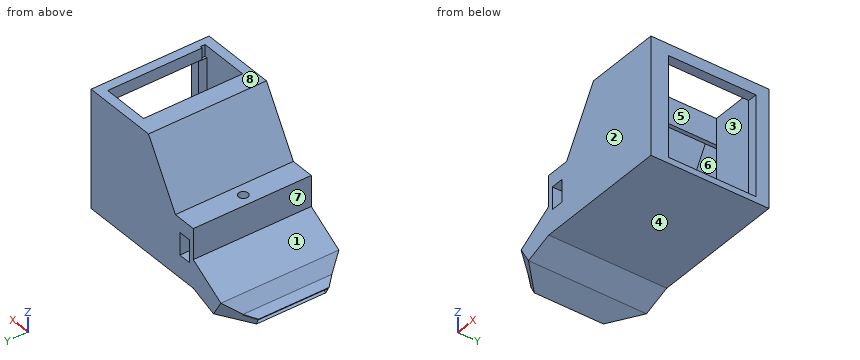
```python
from build123d import *

# Parameters (mm, degrees)
F0_W      = 5.5
F0_H      = 9.5
F1_DEPTH  = 50
F2_T      = -2.5
F3_W      = 46
F3_H      = 4
F4_DEPTH  = 18
F5_DEPTH  = 30
F6_W      = 2
F6_H      = 3
F7_DEPTH  = 42.640873421
F8_W      = 20
F8_H      = 42
F9_DEPTH  = 4.859126579
F10_W     = 1.7037652433
F10_H     = 3.2813884318
F11_DEPTH = 45
F12_W     = 1
F12_H     = 2
F13_DEPTH = 5
F14_DEPTH = 42.640873421
F15_DEPTH = 5
F16_DEPTH = 3
F17_DEPTH = 2
F20_DEPTH = 50
F21_DEPTH = 25
F22_DEPTH = 15
F23_DEPTH = 0.5
F24_DEPTH = 3
F25_DEPTH = 2
F26_R     = 2
F27_DEPTH = 6


with BuildPart() as f1:
    # F0 (on Front) → F1 (new body)
    with BuildSketch(Plane.XZ):
        Polygon((0, 12), (0, 0), (20, 0), (20, 25), (10, 25), (0, 25), align=None)
        with Locations((4.75, 14.25)):
            Rectangle(F0_W, F0_H, mode=Mode.SUBTRACT)
        Polygon((20, 25), (20, 0), (25, 0), (25, 50), (10, 25), align=None)
        Polygon((-11.2763114494, -4.1042417199), (0, 0), (0, 12), (-15.3952030634, 2.7539454948), align=None)
    extrude(amount=F1_DEPTH)

    # F2
    f2_openings = [f1.faces().sort_by_distance(p)[0] for p in [
        (25, -25, 25),
    ]]
    offset(amount=F2_T, openings=f2_openings, kind=Kind.INTERSECTION)

    # F3 (on face) → F4 (cut)
    with BuildSketch(Plane(origin=(-10.0986787248, 0, -6.0650667312), x_dir=(0, -1, 0), z_dir=(-0.8572734018, 0, -0.5148614518))):
        with Locations((25, 6.2872808221)):
            Rectangle(F3_W, F3_H)
    extrude(amount=-F4_DEPTH, mode=Mode.SUBTRACT)

    # F5 (add): a face of the model
    f5_faces = [f1.faces().sort_by_distance(p)[0] for p in [
        (25, -25, 0.7071067812),
    ]]
    extrude(f5_faces, amount=F5_DEPTH)

    # F6 (on face) → F7 (join, through all)
    with BuildSketch(Plane(origin=(0, 0, 45.140873421), x_dir=(1, 0, 0), z_dir=(0, 0, -1))):
        with Locations((54, 46)):
            Rectangle(F6_W, F6_H)
        with Locations((54, 4)):
            Rectangle(F6_W, F6_H)
    extrude(amount=F7_DEPTH)

    # F8 (on face) → F9 (cut, through all)
    with BuildSketch(Plane.XY.offset(50)):
        with Locations((43, -25)):
            Rectangle(F8_W, F8_H)
    extrude(amount=-F9_DEPTH, mode=Mode.SUBTRACT)

    # F10 (on face) → F11 (join, through all)
    with BuildSketch(Plane.XZ.offset(2.5)):
        with Locations((32.1481173784, 43.5001792051)):
            Rectangle(F10_W, F10_H)
    extrude(amount=F11_DEPTH)

    # F12 (on face) → F13 (cut)
    with BuildSketch(Plane.XY.offset(50)):
        with Locations((53.5, -45)):
            Rectangle(F12_W, F12_H)
    extrude(amount=-F13_DEPTH, mode=Mode.SUBTRACT)

    # F14 (add, through all): faces of the model
    f14_faces = [f1.faces().sort_by_distance(p)[0] for p in [
        (43, -46.75, 45.140873421),
        (43, -3.25, 45.140873421),
    ]]
    extrude(f14_faces, amount=F14_DEPTH)

    # F15 (add): a face of the model
    f15_faces = [f1.faces().sort_by_distance(p)[0] for p in [
        (55, -25, 0.7071067812),
    ]]
    extrude(f15_faces, amount=F15_DEPTH)

    # F16 (add): a face of the model
    f16_faces = [f1.faces().sort_by_distance(p)[0] for p in [
        (32.1481173784, -25, 41.8594849892),
    ]]
    extrude(f16_faces, amount=F16_DEPTH)

    # F17 (add): a face of the model
    f17_faces = [f1.faces().sort_by_distance(p)[0] for p in [
        (56.5014165477, -44.5, 23.810402831),
    ]]
    extrude(f17_faces, amount=F17_DEPTH)

    # F19 (on face) → F20 (join)
    with BuildSketch(Plane.XZ.offset(50)):
        Polygon((-11.2763114494, -4.1042417199), (-15.3952030634, 2.7539454948), (-19.6083863192, -2.1957097309), (-23.1083863192, -3.9201829974), (-21.6654660693, -6.8880073104), align=None)
    extrude(amount=-F20_DEPTH)

    # F18 (on face) → F21 (cut)
    with BuildSketch(Plane(origin=(-5.2965243386, 0, 8.819012226), x_dir=(0.8572734018, 0, 0.5148614518), z_dir=(-0.5148614518, 0, 0.8572734018))):
        Polygon((-33.7799977267, -50), (-11.7799977267, -50), (-33.7799977267, -28), align=None)
        Polygon((-33.7799977267, -22), (-11.7799977267, 0), (-33.7799977267, 0), align=None)
    extrude(amount=-F21_DEPTH, mode=Mode.SUBTRACT)

    # F22 (cut): a face of the model
    f22_faces = [f1.faces().sort_by_distance(p)[0] for p in [
        (-22.3892898276, -25, -5.3992335904),
    ]]
    extrude(f22_faces, amount=-F22_DEPTH, mode=Mode.SUBTRACT)

    # F23 (add): a face of the model
    f23_faces = [f1.faces().sort_by_distance(p)[0] for p in [
        (-21.2912627093, -25, -3.0248741153),
    ]]
    extrude(f23_faces, amount=-F23_DEPTH)

    # F24 (cut): a face of the model
    f24_faces = [f1.faces().sort_by_distance(p)[0] for p in [
        (60, -25, 0.7071067812),
    ]]
    extrude(f24_faces, amount=-F24_DEPTH, mode=Mode.SUBTRACT)

    # F25 (add): a face of the model
    f25_faces = [f1.faces().sort_by_distance(p)[0] for p in [
        (6.25, -25, 21.5),
    ]]
    extrude(f25_faces, amount=F25_DEPTH)

    # F26 (on face) → F27 (cut)
    with BuildSketch(Plane.XY.offset(25)):
        with Locations((5, -25)):
            Circle(F26_R)
    extrude(amount=-F27_DEPTH, mode=Mode.SUBTRACT)


solid = f1.part
```
The listing builds one solid part. Answer for the finished solid, in the listing's coordinates (mm). Face numbers are marked on the shaded views. A direction names the side the tool comes from. Coordinates: 2 decimals unless noted, no trailing zeros. Write each loop counter-clockwise with the first axis right and the second up, starting at its lowest first coordinate (ties: lowest second). Pieces come first, ordered by that corner, then holes. Notation, with made-up numbers: (83.5, -25.75) -> (94.5, -25.75) arc R32 cw to (94.5, 11.25) -> close; hole circle Ø10 at (75.5, -6.5). An arc over 180 degrees is marked (long way). Write each question's results on one line, items separated by ' | '. Start each with the question number.
1) For a pull along X with two mould halves and no side action, classify the marked faces 1, 2 and 3 as +X half, -X half, draft (parallel to the pull), parting line (faces both ways), or undercut.
2) Straight lines are drawn through the part: probe 1 along Y at (x, z) = (5, 22); probe 2 along Y at (x, z) = (47, 23.5); probe 3 along Z at (x, y) = (32, -18.5). For each, find the intervals that lie inside material, in ascending order.
3) A cutting plane is placed at B-B (x = 42). Determine the outline of the cut face in (y, z).
4) Flat-ended cylindrical pins translate along their axes: pin 1 Ø1.5 at (y, z) = (-15, 20.5) entering from +X; pin 2 Ø10.5 at (y, z) = (-23, 15.5) entering from -X; pin 3 Ø3 at (x, y) = (3.5, -13.5) entering from +Z. Find the tip coordinate at first contact, or state that the pin passes through.
5) A tool of negligible diameter and unlimited length cuts with its end or side. For the marked faces 4, 5, 6, 7 and 8, from which of +Z, -Z, +X, -X, +Y, -Y can it reach the whole face along a straight path? Write none if from no direction.
6) A cutting plane is placed at C-C (y = -41.5). Count the separate pieces of the cut face and the enclosed holes in it, then the cut area to 3 significant figures.
7) A cutting plane is placed at D-D (x = 20.5). Determine the outline of the cut face in (y, z), then the cut area to 3 significant figures.
8) A cutting plane is placed at A-A (x = 5). Determine the outline of the cut face in (y, z).
Values follow:
1) face 1: -X half | face 2: draft | face 3: undercut
2) probe 1: -50 to -27, -23 to 0 | probe 2: -50 to -46, -4 to 0 | probe 3: 0 to 2.5, 38.86 to 50
3) outline: (-50, 0) -> (0, 0) -> (0, 50) -> (-4, 50) -> (-4, 2.5) -> (-46, 2.5) -> (-46, 50) -> (-50, 50) -> close
4) pin 1: x = 10 | pin 2: x = -2.91 | pin 3: z = 25
5) face 4: -Z, +X, +Y, -Y | face 5: +Z | face 6: none | face 7: +Z, -X, +Y, -Y | face 8: +Z, +X, -X, +Y, -Y
6) separate pieces: 2 | enclosed holes: 1 | area: 516 mm²
7) outline: (-50, 0) -> (0, 0) -> (0, 42.5) -> (-50, 42.5) -> close; hole (-47.5, 2.5) -> (-2.5, 2.5) -> (-2.5, 37.64) -> (-47.5, 37.64) -> close | area: 544 mm²
8) outline: (-50, 0) -> (0, 0) -> (0, 9.5) -> (-50, 9.5) -> close; (-50, 19) -> (-27, 19) -> (-27, 25) -> (-50, 25) -> close; (-23, 19) -> (0, 19) -> (0, 25) -> (-23, 25) -> close; hole (-47.5, 2.5) -> (-2.5, 2.5) -> (-2.5, 7) -> (-47.5, 7) -> close
